Part print with two shaded views. Sizes in mm from the minimum x, y, z corner. A direction names the side the tool comes from. Round coordinates to 2 decimals unless told otherwise and drop trailing zeros. Write each loop counter-clockwise with the first axis right and the second up, starting at its lowest first coordinate (ties: lowest second). Pieces come first, ordered by that corner, then holes. Notation, with made-up numbers: (12, -10.75) -> (57, -10.75) arc R22 cw to (57, 1.25) -> close; hole circle Ø1 at (4.25, 6.5). An arc over 180 degrees is marked (long way). Put each result on its own line as item: value. Start each with the question number.
1. Saw through at D-D on z = 23. List the corners of the cut face in (x, y).
2. Flat gauge pins, fed straight in: P1, Ø7, axis at x = 24, y = 32, coming from the -Z side; P2, Ø2, axis at x = 11.5, y = 39.5, coming from the -Z side. Where does each tip first touch, or does it go through?
3. 3-axis set-ups, long thin cutter, end or side, ignore diameter. For the marked faces 4, 5 and 6: which of +Z, -Z, +X, -X, +Y, -Y reach the whole face in a straight line?
4. Saw through at B-B on y = 32. List the corners of the cut face in (x, z), and give its area (3 significant figures).
5. Saw through at C-C on z = 3.25. List the corners of the cut face in (x, y) (3 decimals), and give its area (3 significant figures).
6. Saw through at A-A on x = 24. List the corners of the cut face in (y, z), and give its area (3 significant figures).
7. Pull direction Z, two halves, no side cores. Call the marked faces 1, 2 and 3: pulls with the +Z half, pulls with the -Z half, needs draft (parallel to the pull), parting line crosses it, or undercut.
8. Drill centre lines: line 1 (Y direction, x = 24, z = 20.5); line 2 (X direction, y = 5, z = 2.75); line 3 (Z direction, x = 66, y = 3). Where is each one in solid material? Low to high. Write a range as from..to.
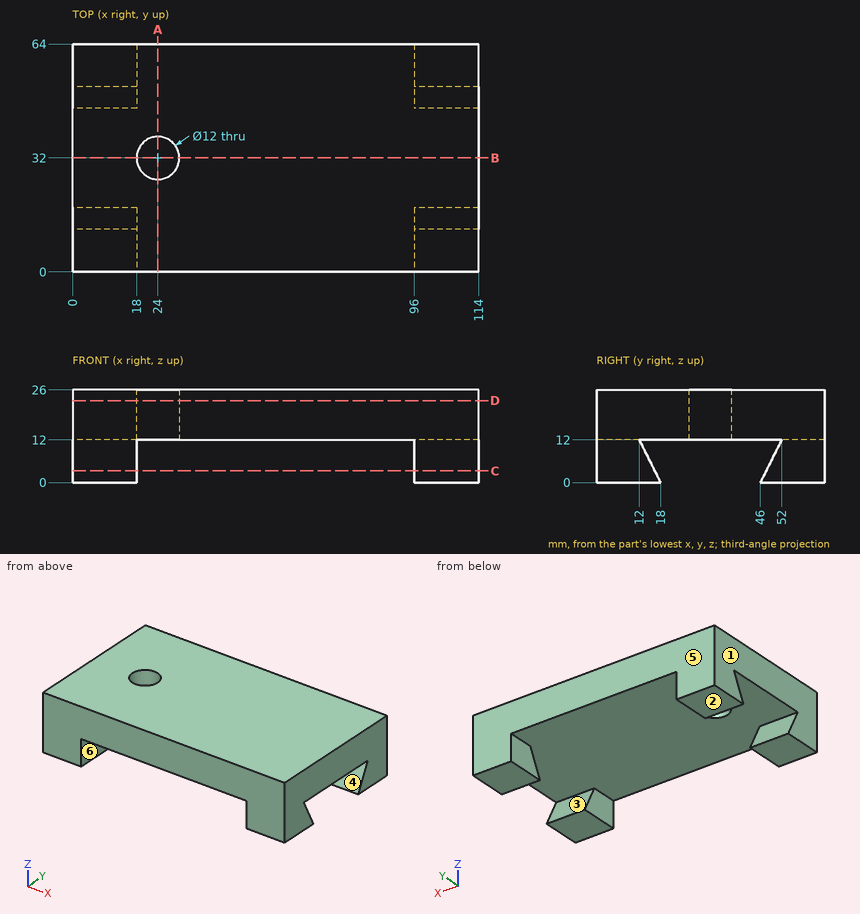
Return value:
1. outline: (0, 0) -> (114, 0) -> (114, 64) -> (0, 64) -> close; hole circle Ø12 at (24, 32)
2. P1: passes through
2. P2: stops at z = 12
3. face 4: +X, -X
3. face 5: +Z, -Z, +X, -X, +Y
3. face 6: -Z, +Y, -Y
4. outline: (0, 12) -> (18, 12) -> (18, 26) -> (0, 26) -> close; (30, 12) -> (114, 12) -> (114, 26) -> (30, 26) -> close
4. area: 1,430 mm^2
5. outline: (0, 0) -> (18, 0) -> (18, 16.375) -> (0, 16.375) -> close; (0, 47.625) -> (18, 47.625) -> (18, 64) -> (0, 64) -> close; (96, 0) -> (114, 0) -> (114, 16.375) -> (96, 16.375) -> close; (96, 47.625) -> (114, 47.625) -> (114, 64) -> (96, 64) -> close
5. area: 1,180 mm^2
6. outline: (0, 12) -> (26, 12) -> (26, 26) -> (0, 26) -> close; (38, 12) -> (64, 12) -> (64, 26) -> (38, 26) -> close
6. area: 728 mm^2
7. face 1: needs draft
7. face 2: pulls with the -Z half
7. face 3: undercut
8. line 1: y = 0..26, 38..64
8. line 2: x = 0..18, 96..114
8. line 3: z = 12..26
